Verification items for this drawing (mm, ordinates from the low corner). Round coordinates to 2 decimals unless told otherwise and drop trailing zeros. Order: outer loops, then holes, each group sorted by start corner. A loop starts at its lowest first (then second) coordinate and runs counter-clockwise, first axis right, second up.
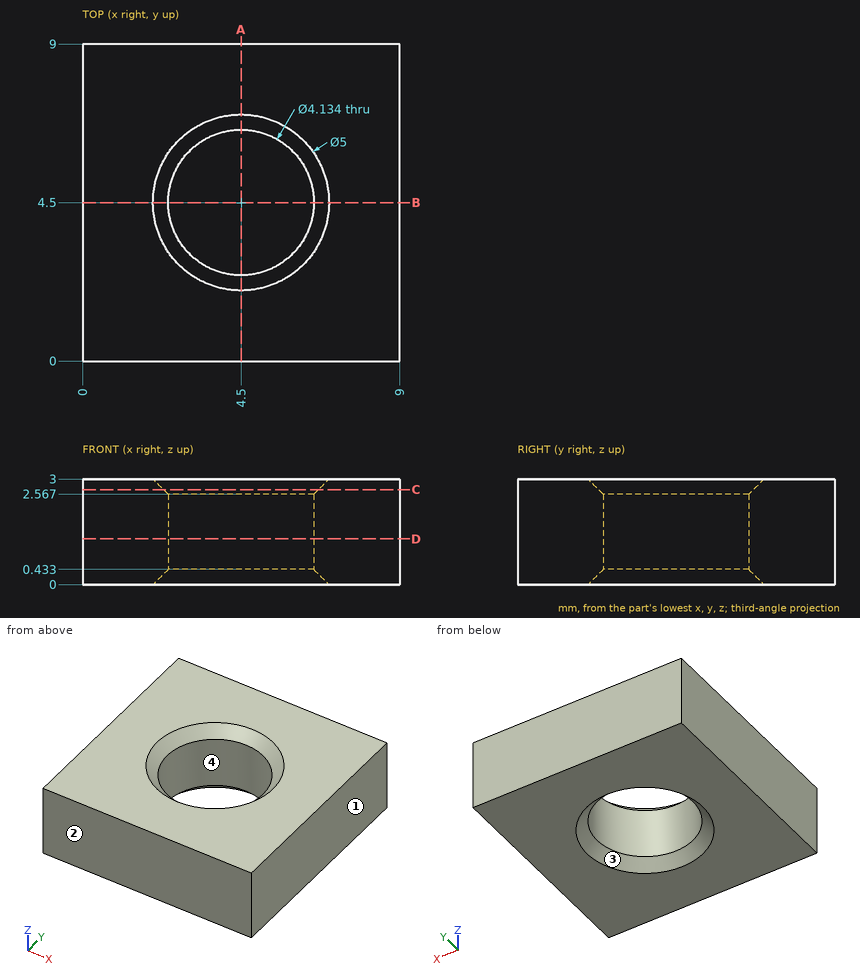
Item 1: Sectioned sample at A-A (x = 4.5). Record the cut outline in (y, z).
Answer:
outline: (0, 0) - (2, 0) - (2.43, 0.43) - (2.43, 2.57) - (2, 3) - (0, 3) - close; (6.57, 0.43) - (7, 0) - (9, 0) - (9, 3) - (7, 3) - (6.57, 2.57) - close
Item 2: Release check for a two-part mould opening along Y. For the marked faces 1, 2, 3 and 4 record: released by +Y, released by -Y, zero draft, split by the parting line, or undercut.
Answer:
face 1: zero draft
face 2: released by -Y
face 3: undercut
face 4: undercut
Item 3: Scan lines: line 1 along X through (y, z) = (4.5, 1.45); line 2 along Y through (x, z) = (5, 2.9); line 3 along Y through (x, z) = (4, 1.45). Record each from-to range of solid material in increasing order.
Answer:
line 1: x = 0 to 2.43, 6.57 to 9
line 2: y = 0 to 2.15, 6.85 to 9
line 3: y = 0 to 2.49, 6.51 to 9
Item 4: Sectioned sample at D-D (z = 1.3). Record the cut outline in (x, y).
Answer:
outline: (0, 0) - (9, 0) - (9, 9) - (0, 9) - close; hole circle Ø4.13 at (4.5, 4.5)
Item 5: Sectioned sample at C-C (z = 2.7). Record the cut outline in (x, y), and give its area (3 significant figures).
Answer:
outline: (0, 0) - (9, 0) - (9, 9) - (0, 9) - close; hole circle Ø4.4 at (4.5, 4.5)
area: 65.8 mm2
Item 6: Go/stop test with flat-tipped pins: P1, Ø1, axis at y = 4.5, z = 1, coming from the -X side; P2, Ø3.5, axis at x = 4.5, y = 4.5, coming from the +Z side. Record where each tip stops, or that it passes through.
Answer:
P1: stops at x = 0
P2: passes through
